from build123d import *

# Parameters (mm, degrees)
F1_DEPTH = 12.7


with BuildPart() as f1:
    # F0 (on Front) → F1 (new body)
    with BuildSketch(Plane.XZ):
        with BuildLine():
            Line((0, 79.375), (0, 89.5573869348))
            Line((0, 89.5573869348), (0, 100.0252))
            Line((0, 100.0252), (-0.0357827719, 100.0252))
            ThreePointArc((-0.0357827719, 100.0252), (-1.6439653205, 97.2637315367), (-4.8393784091, 97.2997089891))
            Line((-4.8393784091, 97.2997089891), (-4.8393784091, 78.6193928983))
            ThreePointArc((-4.8393784091, 78.6193928983), (-2.4490062004, 79.1849607469), (0, 79.375))
        make_face()
        with BuildLine():
            Line((0, 100.0252), (0, 89.5573869348))
            Line((0, 89.5573869348), (0, 79.375))
            ThreePointArc((0, 79.375), (10.5003255158, 75.40625), (15.7504882737, 65.484375))
            Line((15.7504882737, 65.484375), (9.4502929642, 115.490625))
            ThreePointArc((9.4502929642, 115.490625), (9.5063048942, 114.896483242), (9.525, 114.3))
            ThreePointArc((9.525, 114.3), (6.7351920908, 107.5648079092), (0, 104.775))
            Line((0, 104.775), (0, 100.0252))
        make_face()
        with BuildLine():
            Line((-0.0357827719, 100.0252), (0, 100.0252))
            Line((0, 100.0252), (0, 104.775))
            ThreePointArc((0, 104.775), (-7.1202192788, 107.9732233782), (-9.4589053806, 115.4201490977))
            Line((-9.4589053806, 115.4201490977), (-14.9877324754, 68.7329246359))
            ThreePointArc((-14.9877324754, 68.7329246359), (-11.0776416797, 74.8710808553), (-4.8393784091, 78.6193928983))
            Line((-4.8393784091, 78.6193928983), (-4.8393784091, 97.2997089891))
            ThreePointArc((-4.8393784091, 97.2997089891), (-4.7776002233, 102.7866684633), (-0.0357827719, 100.0252))
        make_face()
        with BuildLine():
            ThreePointArc((15.7504882737, 65.484375), (10.5003255158, 75.40625), (0, 79.375))
            Line((0, 79.375), (0, 66.675))
            ThreePointArc((0, 66.675), (2.2450640303, 65.7450640303), (3.175, 63.5))
            ThreePointArc((3.175, 63.5), (2.2450640303, 61.2549359697), (0, 60.325))
            Line((0, 60.325), (0, 47.625))
            ThreePointArc((0, 47.625), (10.6492737428, 51.7267849017), (15.7954255641, 61.9125))
            ThreePointArc((15.7954255641, 61.9125), (15.8550939106, 62.7052534459), (15.875, 63.5))
            ThreePointArc((15.875, 63.5), (15.8438414904, 64.4941387366), (15.7504882737, 65.484375))
        make_face()
        with BuildLine():
            Line((0, 66.675), (0, 79.375))
            ThreePointArc((0, 79.375), (-2.4490062004, 79.1849607469), (-4.8393784091, 78.6193928983))
            ThreePointArc((-4.8393784091, 78.6193928983), (-11.0776416797, 74.8710808553), (-14.9877324754, 68.7329246359))
            Line((-14.9877324754, 68.7329246359), (-15.7954255641, 61.9125))
            ThreePointArc((-15.7954255641, 61.9125), (-10.6492737428, 51.7267849017), (0, 47.625))
            Line((0, 47.625), (0, 60.325))
            ThreePointArc((0, 60.325), (-3.175, 63.5), (0, 66.675))
        make_face()
        with BuildLine():
            ThreePointArc((-9.4589053806, 115.4201490977), (-7.1202192788, 107.9732233782), (0, 104.775))
            ThreePointArc((0, 104.775), (6.7351920908, 107.5648079092), (9.525, 114.3))
            ThreePointArc((9.525, 114.3), (9.5063048942, 114.896483242), (9.4502929642, 115.490625))
            ThreePointArc((9.4502929642, 115.490625), (-0.0355000934, 123.8249338446), (-9.4589053806, 115.4201490977))
        make_face()
        with BuildLine():
            ThreePointArc((3.175, 114.3), (2.2450640303, 112.0549359697), (0, 111.125))
            ThreePointArc((0, 111.125), (-2.2450640303, 116.5450640303), (3.175, 114.3))
        make_face(mode=Mode.SUBTRACT)
        with BuildLine():
            ThreePointArc((15.7954255641, 61.9125), (10.6492737428, 51.7267849017), (0, 47.625))
            Line((0, 47.625), (0, 9.525))
            ThreePointArc((0, 9.525), (6.7351920908, 6.7351920908), (9.525, 0))
            Line((9.525, 0), (36.5125, 0))
            ThreePointArc((36.5125, 0), (38.9384772185, 5.7120069047), (44.7334821429, 7.9324362036))
            Line((44.7334821429, 7.9324362036), (18.9676000005, 8.8532337108))
            ThreePointArc((18.9676000005, 8.8532337108), (13.2611998974, 11.5713591498), (11.3411865923, 17.5933818124))
            Line((11.3411865923, 17.5933818124), (15.7954255641, 61.9125))
        make_face()
        with BuildLine():
            Line((0, 9.525), (0, 47.625))
            ThreePointArc((0, 47.625), (-10.6492737428, 51.7267849017), (-15.7954255641, 61.9125))
            Line((-15.7954255641, 61.9125), (-9.4772553384, -0.9525))
            ThreePointArc((-9.4772553384, -0.9525), (-7.063929059, 6.3895642457), (0, 9.525))
        make_face()
        with BuildLine():
            ThreePointArc((9.525, 0), (6.7351920908, 6.7351920908), (0, 9.525))
            Line((0, 9.525), (0, 3.175))
            ThreePointArc((0, 3.175), (2.2450640303, 2.2450640303), (3.175, 0))
            Line((3.175, 0), (9.525, 0))
        make_face()
        with BuildLine():
            Line((0, 3.175), (0, 9.525))
            ThreePointArc((0, 9.525), (-7.063929059, 6.3895642457), (-9.4772553384, -0.9525))
            ThreePointArc((-9.4772553384, -0.9525), (-6.2623833816, -7.1769199091), (0.3401785714, -9.5189234444))
            ThreePointArc((0.3401785714, -9.5189234444), (6.8544082857, -6.6138273378), (9.525, 0))
            Line((9.525, 0), (3.175, 0))
            ThreePointArc((3.175, 0), (-2.2450640303, -2.2450640303), (0, 3.175))
        make_face()
        with BuildLine():
            Line((36.5125, 0), (9.525, 0))
            ThreePointArc((9.525, 0), (6.8544082857, -6.6138273378), (0.3401785714, -9.5189234444))
            Line((0.3401785714, -9.5189234444), (44.7334821429, -7.9324362036))
            ThreePointArc((44.7334821429, -7.9324362036), (38.9384772185, -5.7120069047), (36.5125, 0))
        make_face()
        with BuildLine():
            ThreePointArc((44.7334821429, 7.9324362036), (38.9384772185, 5.7120069047), (36.5125, 0))
            ThreePointArc((36.5125, 0), (38.9384772185, -5.7120069047), (44.7334821429, -7.9324362036))
            ThreePointArc((44.7334821429, -7.9324362036), (50.1620069047, -5.5115227815), (52.3875, 0))
            ThreePointArc((52.3875, 0), (50.1620069047, 5.5115227815), (44.7334821429, 7.9324362036))
        make_face()
        with BuildLine():
            ThreePointArc((47.625, 0), (44.45, -3.175), (41.275, 0))
            ThreePointArc((41.275, 0), (44.45, 3.175), (47.625, 0))
        make_face(mode=Mode.SUBTRACT)
    extrude(amount=F1_DEPTH)


solid = f1.part
Geometry: final body of the model. Coordinates: model frame, mm. A direction names the side the tool comes from. Round coordinates to 2 decimals unless told otherwise and drop trailing zeros. Loops run counter-clockwise (first coordinate to the right, second up) from the corner with the lowest first, then second, coordinate; pieces in that order, holes last. Notation, with made-up numbers: M -28.75,64.5 L -5.75,64.5 A23 cw -5.75,97.5 Z; hole C -22,71 d8. An arc over 180 degrees is marked long. One line per question, with ' | ' between items.
(1) Pull-direction query (Z, two-part tool) for faces 1 (the cylindrical face through (-6.34, -6.26, -7.11)), 2 (the flat face through (12.644, -6.261, 90.137)), 3 (the flat face through (13.537, -6.261, 39.443)), 4 (the flat face through (3, 0, 43)); classes: +Z half, -Z half, draft (parallel to the pull), parting line (faces both ways), or undercut.
Check result:
face 1: -Z half | face 2: +Z half | face 3: undercut | face 4: draft
(2) Material intervals for line 1 along Z through (x, y) = (2.5, -4.25); line 2 along Z through (x, y) = (44.45, -3) (3 decimals); line 3 along Z through (x, y) = (-2, -6.75), sorted ascending. Write a range as from..to.
Check result:
line 1: z = -9.44..-1.96, 1.96..61.54, 65.46..112.34, 116.26..123.49 | line 2: z = -7.943..-3.175, 3.175..7.943 | line 3: z = -9.31..-2.47, 2.47..61.03, 65.97..97.09, 102.96..111.83, 116.77..123.61
(3) Access query for faces 5 (the cylindrical face through (13.321, -6.261, 11.503)), 6 (the cylindrical face through (41.52, -6.26, -1.22)). Directions: +Z, -Z, +X, -X, +Y, -Y. A direction counts if a zero-diameter tool reaches every point of the face in a straight line with its end or side. Return the directions, or none.
Check result:
face 5: +X, +Y, -Y | face 6: +Y, -Y
(4) Cut plane A-A on y = -10.5. Give the number of separate pieces and of enclosed holes in the cut face, plus the area to 3 significant figures.
Check result:
separate pieces: 1 | enclosed holes: 5 | area: 3,760 mm2
(5) Contact query for flat-ended pins moving along their axis: P1, Ø5, axis at x = 31, y = -9, coming from the -Z side; P2, Ø3, axis at x = 4, y = -4, coming from the +Z side; P3, Ø5, axis at x = 14.5, z = 106.5, coming from the +Y side; P4, Ø5, axis at x = 28.5, y = -5, coming from the -Z side. Output: stop coordinate, or through.
Check result:
P1: stops at z = -8.51 | P2: stops at z = 123.49 | P3: passes through | P4: stops at z = -8.6
(6) Cut plane C-C on x = 33. Return the cut outline in (y, z), plus the area to 3 significant figures.
Check result:
outline: M -12.7,-8.35 L 0,-8.35 L 0,8.35 L -12.7,8.35 Z | area: 212 mm2
(7) Cut plane D-D on x = 24.5. Return the cut outline in (y, z).
Check result:
outline: M -12.7,-8.66 L 0,-8.66 L 0,8.66 L -12.7,8.66 Z
(8) Cut plane B-B on x = 13.5. Return the cut outline in (y, z).
Check result:
outline: M -12.7,-9.05 L 0,-9.05 L 0,11.31 L -12.7,11.31 Z; M -12.7,39.07 L 0,39.07 L 0,83.35 L -12.7,83.35 Z
